The listing builds one solid part. Answer for the finished solid, in the listing's coordinates (mm). Face numbers are marked on the shaded views. A direction names the side the tool comes from. Round coordinates to 2 decimals unless told otherwise and drop trailing zeros. Write each loop counter-clockwise with the first axis right and the second up, starting at its lowest first coordinate (ties: lowest second). Pieces come first, ordered by that corner, then holes.
Item 1: Find section D-D on z = -15.5. Give the vertices of the cut face in (x, y) (1 decimal).
Item 2: Find section A-A on x = 11.75. Give the vertices of the cut face in (y, z) (1 decimal).
Item 3: A tool of negligible diameter and unlimited length cuts with its end or side. For the marked faces 1, 2, 3, 4 and 5, from which of +Z, -Z, +X, -X, +Y, -Y can it reach the whole face along a straight path? Write none if from no direction.
Item 4: For a pull along Z with two mould halves and no side action, classify the marked faces 6, 7, 8 and 9 as +Z half, -Z half, draft (parallel to the pull), parting line (faces both ways), or undercut.
Item 5: Find the intervals of material crossed by probe 1 along X at (y, z) = (12.7, -2.1) (3 decimals); probe 2 along X at (y, z) = (4.2, -12.7) (3 decimals), in increasing order.
Item 6: Find section C-C on x = 21. Give the vertices of the cut face in (y, z) (3 decimals).
Item 7: Each of these flat-tipped pins is pushed along its axis until it touches: pin 1 (5.5 mm diameter, centred on x = 16.5, z = -9.5, fed in from -Y) (3 decimals); pin 2 (7 mm diameter, centred on y = 18.5, z = -14, fed in from -X); pin 3 (5.5 mm diameter, centred on x = 9, y = 9, fed in from +Z) (3 decimals). Where does it stop, or does it pass through?
Autodesk Inventor part; units mm, degrees
ref_plane "YZ Plane" through (0, 0, 0) normal (1, 0, 0) x (0, 1, 0)
ref_plane "XZ Plane" through (0, 0, 0) normal (0, 1, 0) x (-1, 0, 0)
ref_plane "XY Plane" through (0, 0, 0) normal (0, 0, 1) x (1, 0, 0)
sketch "Sketch1" plane through (0, 0, 0) normal (0, 1, 0) x (-1, 0, 0)
  line L0 (0, 0) -> (-25.4, 0)
  line L1 (-25.4, 0) -> (-25.4, -25.4)
  line L2 (-25.4, -25.4) -> (0, -25.4)
  line L3 (0, -25.4) -> (0, 0)
  line L4 (0, 0) -> (-25.4, -25.4) construction
  line L5 (-25.4, 0) -> (0, -25.4) construction
  circle A0 centre (-12.7, -12.7) radius 9.525
  dimension "d0" = 25.4
  dimension "d1" = 25.4
  dimension "d3" = 19.05
extrude "Extrusion1" add sketch "Sketch1" along normal blind 3.175
sketch "Sketch2" plane through (0, 3.175, 0) normal (0, 1, 0) x (1, 0, 0)
  line L0 (25.4, 25.4) -> (0, 25.4)
  line L1 (0, 0) -> (25.4, 0)
  line L2 (25.4, 0) -> (25.4, 25.4)
  line L3 (25.4, 25.4) -> (0, 25.4)
  line L4 (0, 25.4) -> (0, 0)
  line L5 (0, 25.4) -> (0, 0) construction
  line L6 (0, 0) -> (25.4, 25.4) construction
  line L7 (0, 25.4) -> (25.4, 0) construction
  circle A0 centre (12.7, 12.7) radius 3.175
  dimension "d39" = 6.35
extrude "Extrusion2" add sketch "Sketch2" along normal blind 4.7625
sketch "Sketch4" plane through (0, 0, 0) normal (0, 0, 1) x (1, 0, 0)
  line L0 (0, 0) -> (0, 7.9375)
  line L1 (0, 0) -> (25.4, 0)
  line L2 (25.4, 0) -> (25.4, 25.4)
  line L3 (25.4, 25.4) -> (0, 25.4)
  line L4 (0, 25.4) -> (0, 0)
  line L5 (0, 25.4) -> (25.4, 0) construction
  line L6 (25.4, 25.4) -> (0, 0) construction
  circle A0 centre (12.7, 12.7) radius 9.525
  dimension "d13" = 25.4
  dimension "d14" = 25.4
  dimension "d15" = 19.05
extrude "Extrusion4" add sketch "Sketch4" against normal blind 3.175
sketch "Sketch5" plane through (0, 0, 0) normal (0, 0, 1) x (1, 0, 0)
  line L0 (0, 0) -> (0, 25.4) construction
  line L1 (0, 0) -> (25.4, 0) construction
  line L2 (0, 25.4) -> (25.4, 0) construction
  line L3 (0, 25.4) -> (25.4, 25.4) construction
  line L4 (25.4, 0) -> (25.4, 25.4) construction
  line L5 (0, 0) -> (0, 7.9375) construction
  line L6 (25.4, 25.4) -> (0, 0) construction
  circle A0 centre (12.7, 12.7) radius 9.525
  dimension "d18" = 19.05
extrude "Extrusion5" cut sketch "Sketch5" against normal blind 3.175
sketch "Sketch6" plane through (0, 0, -3.175) normal (0, 0, -1) x (-1, 0, 0)
  line L0 (-25.4, 0) -> (-25.4, 25.4)
  line L1 (-25.4, 25.4) -> (0, 25.4)
  line L2 (0, 25.4) -> (0, 0)
  line L3 (0, 0) -> (-25.4, 0)
  line L4 (-25.4, 0) -> (-25.4, 25.4)
  line L5 (0, 0) -> (0, 25.4) construction
  line L6 (-25.4, 25.4) -> (0, 0) construction
  line L7 (0, 0) -> (0, 25.4) construction
  line L8 (0, 25.4) -> (-25.4, 0) construction
  circle A0 centre (-12.7, 12.7) radius 3.175
  dimension "d40" = 6.35
extrude "Extrusion6" add sketch "Sketch6" along normal blind 4.7625
sketch "Sketch7" plane through (25.4, 0, 0) normal (1, 0, 0) x (0, 0, -1)
  line L0 (0, 25.4) -> (7.9375, 25.4)
  line L1 (25.4, 0) -> (25.4, 7.9375)
  line L2 (0, 25.4) -> (25.4, 25.4)
  line L3 (25.4, 25.4) -> (25.4, 0)
  line L4 (25.4, 0) -> (0, 0)
  line L5 (0, 0) -> (0, 25.4)
  line L6 (0, 25.4) -> (25.4, 0) construction
  line L7 (25.4, 25.4) -> (0, 0) construction
  circle A0 centre (12.7, 12.7) radius 9.525
  dimension "d24" = 19.05
extrude "Extrusion7" add sketch "Sketch7" against normal blind 3.175
sketch "Sketch8" plane through (25.4, 0, 0) normal (1, 0, 0) x (0, 0, -1)
  line L0 (0, 0) -> (0, 25.4) construction
  line L1 (0, 0) -> (25.4, 0) construction
  line L2 (0, 25.4) -> (25.4, 0) construction
  line L3 (25.4, 0) -> (25.4, 25.4) construction
  line L4 (25.4, 25.4) -> (0, 0) construction
  circle A0 centre (12.7, 12.7) radius 9.525
  dimension "d27" = 19.05
extrude "Extrusion8" cut sketch "Sketch8" against normal blind 3.175
sketch "Sketch9" plane through (22.225, 0, 0) normal (-1, 0, 0) x (0, 0, 1)
  line L0 (-25.4, 25.4) -> (-25.4, 7.9375)
  line L1 (-25.4, 25.4) -> (0, 25.4)
  line L2 (0, 25.4) -> (0, 0)
  line L3 (0, 0) -> (-25.4, 0)
  line L4 (-25.4, 0) -> (-25.4, 25.4)
  line L5 (-25.4, 0) -> (0, 0) construction
  line L6 (-25.4, 25.4) -> (0, 0) construction
  line L7 (0, 0) -> (0, 25.4) construction
  line L8 (0, 25.4) -> (-25.4, 0) construction
  circle A0 centre (-12.7, 12.7) radius 3.175
  dimension "d41" = 6.35
extrude "Extrusion9" add sketch "Sketch9" along normal blind 4.7625
sketch "Sketch10" plane through (0, 0, 0) normal (0, -1, 0) x (1, 0, 0)
  line L0 (0, -25.4) -> (0, -7.9375)
  line L1 (25.4, 0) -> (0, 0)
  line L2 (0, -25.4) -> (25.4, -25.4)
  line L3 (25.4, -25.4) -> (25.4, 0)
  line L4 (25.4, 0) -> (0, 0)
  line L5 (0, 0) -> (0, -25.4)
  line L6 (17.4625, -25.4) -> (0, -25.4) construction
  line L7 (25.4, 0) -> (25.4, -25.4) construction
  line L8 (0, -25.4) -> (25.4, 0) construction
  line L9 (25.4, 0) -> (0, 0) construction
  line L10 (0, -25.4) -> (0, 0) construction
  line L11 (0, 0) -> (25.4, -25.4) construction
  circle A0 centre (12.7, -12.7) radius 9.525
  dimension "d33" = 19.05
extrude "Extrusion10" cut sketch "Sketch10" against normal blind 3.175 contours A0
sketch "Sketch11" plane through (0, 0, 0) normal (0, 0, 1) x (1, 0, 0)
  line L0 (0, 7.9375) -> (0, 25.4) construction
  line L1 (25.4, 0) -> (25.4, 25.4) construction
  line L2 (0, 25.4) -> (25.4, 0) construction
  line L3 (25.4, 0) -> (25.4, 25.4) construction
  line L4 (25.4, 25.4) -> (0, 0) construction
  circle A0 centre (12.7, 12.7) radius 9.525
  dimension "d36" = 19.05
extrude "Extrusion11" cut sketch "Sketch11" against normal blind 3.175
sketch "Sketch12" plane through (0, 0, 0) normal (0, 0, 1) x (1, 0, 0)
  line L0 (12.7, 22.3828) -> (25.4, 22.3828) construction
  line L1 (0, 25.4) -> (17.4625, 25.4)
  line L2 (25.4, 22.3828) -> (14.2875, 22.3828)
  line L3 (14.2875, 22.3828) -> (14.2875, 25.4)
  line L4 (14.2875, 25.4) -> (25.4, 25.4)
  line L5 (25.4, 25.4) -> (25.4, 22.3828)
  point P0 (0, 0)
  dimension "d42" = 11.1125
extrude "Extrusion12" cut sketch "Sketch12" against normal blind 25.4
sketch "Sketch13" plane through (0, 0, 0) normal (0, -1, 0) x (1, 0, 0)
  line L0 (17.4625, -25.4) -> (25.4, -25.4)
  line L1 (25.4, -25.4) -> (14.2875, -25.4)
  line L2 (14.2875, -25.4) -> (14.2875, -22.3774)
  line L3 (14.2875, -22.3774) -> (25.4, -22.3774)
  line L4 (25.4, -22.3774) -> (25.4, -25.4)
  point P0 (0, 0)
  dimension "d45" = 11.1125
  dimension "d46" = 3.0226
extrude "Extrusion13" cut sketch "Sketch13" against normal blind 25.4
properties part number "MountingBracket_4"
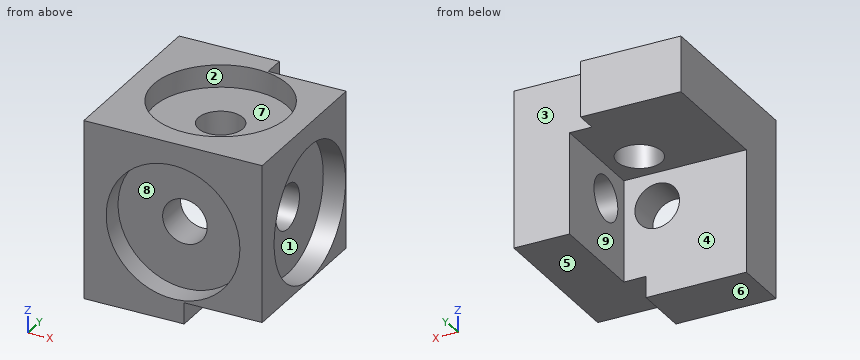
Check values:
1. outline: (0, 0) - (3.6, 0) - (3.6, 3.2) - (11.2, 3.2) - (11.2, 7.9) - (0, 7.9) - close; (14.2, 3.2) - (21.8, 3.2) - (21.8, 0) - (25.4, 0) - (25.4, 3.6) - (22.2, 3.6) - (22.2, 11.2) - (17.5, 11.2) - (17.5, 7.9) - (14.2, 7.9) - close; (17.5, 14.2) - (22.2, 14.2) - (22.2, 21.8) - (25.4, 21.8) - (25.4, 22.4) - (17.5, 22.4) - close
2. outline: (0, -25.4) - (7.9, -25.4) - (7.9, -15.7) - (3.2, -15.7) - (3.2, -22.2) - (0, -22.2) - close; (0, -3.2) - (3.2, -3.2) - (3.2, -9.7) - (7.9, -9.7) - (7.9, -7.9) - (9.7, -7.9) - (9.7, -3.2) - (3.2, -3.2) - (3.2, 0) - (0, 0) - close; (15.7, -7.9) - (25.4, -7.9) - (25.4, 0) - (22.2, 0) - (22.2, -3.2) - (15.7, -3.2) - close
3. face 1: +X
3. face 2: +Z
3. face 3: +Z, -Z, +X, +Y
3. face 4: -Z, -X, +Y
3. face 5: -Z, +X, +Y, -Y
4. face 6: -Z half
4. face 7: +Z half
4. face 8: undercut
4. face 9: draft
5. probe 1: x = 0 to 3.175, 22.225 to 25.4
5. probe 2: x = 0 to 9.525, 15.875 to 22.225
6. outline: (0, -22.377) - (22.383, -22.377) - (22.383, 0) - (17.373, 0) - (17.373, -3.175) - (8.027, -3.175) - (8.027, 0) - (0, 0) - (0, -8.027) - (3.175, -8.027) - (3.175, -17.373) - (0, -17.373) - close; hole circle Ø6.35 at (12.7, -12.7)
7. pin 1: stops at y = 3.175
7. pin 2: stops at x = 17.46
7. pin 3: stops at z = -3.175
